The figure shows three views and two pictorial views of one solid part (mm, origin at its lowest corner). Answer the questions. Coordinates: 2 decimals unless noted, no trailing zeros. Loops run counter-clockwise (first coordinate to the right, second up) from the corner with the lowest first, then second, coordinate; pieces in that order, holes last. Notation, with made-up numbers: (26, -38) - (32, -38) arc R29 cw to (32, -5) - close; hole circle Ø2 at (4, 65). An arc over 180 degrees is marked (long way). One line per question, with ' | ' between items.
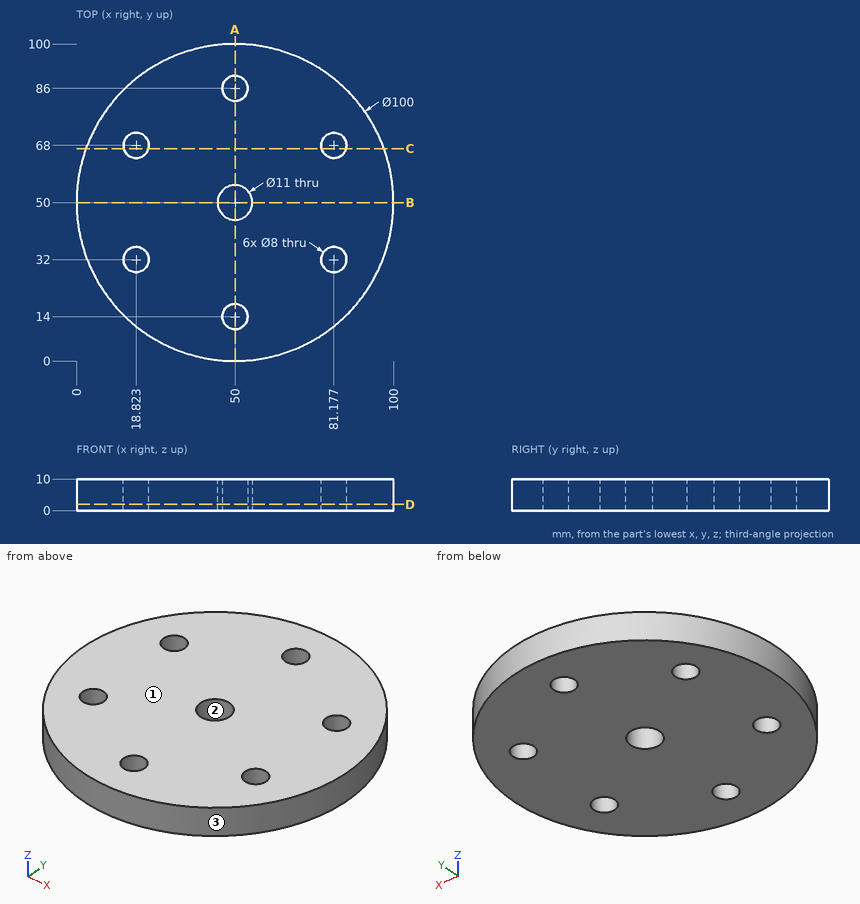
Item 1: Find section B-B, the plane y = 50. Write down the section's boundary in (x, z).
Taken from the geometry:
outline: (0, 0) - (44.5, 0) - (44.5, 10) - (0, 10) - close; (55.5, 0) - (100, 0) - (100, 10) - (55.5, 10) - close
Item 2: Find section C-C, the plane y = 67. Write down the section's boundary in (x, z).
Taken from the geometry:
outline: (2.98, 0) - (14.95, 0) - (14.95, 10) - (2.98, 10) - close; (22.7, 0) - (77.3, 0) - (77.3, 10) - (22.7, 10) - close; (85.05, 0) - (97.02, 0) - (97.02, 10) - (85.05, 10) - close
Item 3: Find section D-D, the plane z = 2. Write down the section's boundary in (x, y).
Taken from the geometry:
outline: circle Ø100 at (50, 50); hole circle Ø8 at (18.82, 32); hole circle Ø8 at (18.82, 68); hole circle Ø11 at (50, 50); hole circle Ø8 at (50, 14); hole circle Ø8 at (50, 86); hole circle Ø8 at (81.18, 32); hole circle Ø8 at (81.18, 68)
Item 4: Find section A-A, the plane x = 50. Write down the section's boundary in (y, z), plus the area to 3 significant figures.
Taken from the geometry:
outline: (0, 0) - (10, 0) - (10, 10) - (0, 10) - close; (18, 0) - (44.5, 0) - (44.5, 10) - (18, 10) - close; (55.5, 0) - (82, 0) - (82, 10) - (55.5, 10) - close; (90, 0) - (100, 0) - (100, 10) - (90, 10) - close | area: 730 mm2
Item 5: Find the intervals of material crossed by line 1 (Y direction, x = 50, z = 8.5); line 2 (X direction, y = 64.5, z = 8); line 3 (Y direction, x = 18, z = 3.75), in increasing order. Write a range as [from, to].
Taken from the geometry:
line 1: y = [0, 10], [18, 44.5], [55.5, 82], [90, 100] | line 2: x = [2.15, 16.89], [20.76, 79.24], [83.11, 97.85] | line 3: y = [11.58, 28.09], [35.91, 64.09], [71.91, 88.42]
Item 6: The mould has two halves that part along Y. Classify the marked faces 1, 2 and 3: pulls with the +Y half, pulls with the -Y half, needs draft (parallel to the pull), parting line crosses it, or undercut.
Taken from the geometry:
face 1: needs draft | face 2: undercut | face 3: parting line crosses it
Item 7: Each of these flat-tipped pins is pushed along its axis until it touches: pin 1 Ø4 at (y, z) = (65, 9) entering from -X; pin 2 Ø6.5 at (x, y) = (50, 14) entering from -Z; pin 3 Ø3 at (x, z) = (70, 8) entering from -Y; pin 4 Ø2 at (x, z) = (21, 1.5) entering from -Y. Where does it stop, or does it pass through?
Taken from the geometry:
pin 1: stops at x = 1.72 | pin 2: passes through | pin 3: stops at y = 3.55 | pin 4: stops at y = 8.58
